Can you work these out from the model? Positions are in its coordinate system, mm. A direction names the side the tool comes from. Round coordinates to 2 decimals unless told otherwise and drop trailing zeros. Loops run counter-clockwise (first coordinate to the right, second up) from the corner with the lowest first, then second, coordinate; pieces in that order, holes last. Notation, with made-up numbers: M 47,60.25 L 85,60.25 A12 ccw 85,68.25 Z; hole C -2.75,46.25 d9. An arc over 180 degrees is marked long. Return JSON: item names as keys, results as strings.
```python
from build123d import *

# Parameters (mm, degrees)
SKETCH3_W                       = 80
SKETCH3_H                       = 80
SKETCH3_W_2                     = 60
SKETCH3_H_2                     = 60
BOSS_EXTRUDE2_DEPTH             = 1550
SKETCH7_W                       = 60
SKETCH7_H                       = 60
BOSS_EXTRUDE3_DEPTH             = 5
BOSS_EXTRUDE4_REACH             = 1561.207
SKETCH8_W                       = 60
SKETCH8_H                       = 5
BOSS_EXTRUDE4_DIRECTION_2_REACH = 1561.207
CUT_EXTRUDE1_REACH              = 1562.929
CUT_EXTRUDE2_REACH              = 1562.929
FILLET1_R                       = 5
MIRROR1_START                   = -90
MIRROR1_DEPTH                   = 10
MIRROR1_2_DEPTH                 = 10
MIRROR1_START_2                 = -80
MIRROR1_3_OUTLINE_W             = 5
MIRROR1_3_OUTLINE_H             = 25
MIRROR1_3_DEPTH                 = 80
MIRROR1_START_3                 = 10
MIRROR1_4_DEPTH                 = 31.124
MIRROR1_START_4                 = -119.452
MIRROR1_5_DEPTH                 = 29.452
MIRROR1_START_5                 = -140
MIRROR1_6_DEPTH                 = 200
MIRROR1_7_DEPTH                 = 5
FILLET1_OF_MIRROR2_R            = 5


with BuildPart() as part:
    # Sketch3 → Boss-Extrude2 (new body)
    with BuildSketch(Plane(origin=(0, 0, 0), x_dir=(0, 0, -1), z_dir=(1, 0, 0))):
        with Locations((40, 40)):
            Rectangle(SKETCH3_W, SKETCH3_H)
        with Locations((40, 40)):
            Rectangle(SKETCH3_W_2, SKETCH3_H_2, mode=Mode.SUBTRACT)
    extrude(amount=BOSS_EXTRUDE2_DEPTH)

    # Sketch7 → Boss-Extrude3 (add)
    with BuildSketch(Plane(origin=(1535, 0, 0), x_dir=(0, 0, -1), z_dir=(1, 0, 0))):
        Polygon((-60, 95), (140, 95), (140, 15), (90, -25), (-10, -25), (-60, 15), align=None)
        with Locations((40, 40)):
            Rectangle(SKETCH7_W, SKETCH7_H, mode=Mode.SUBTRACT)
    boss_extrude3 = extrude(amount=BOSS_EXTRUDE3_DEPTH)

    # Boss-Extrude4: up to this face of the body (flat: up to its plane)
    boss_extrude4_end = Plane(part.part.faces().sort_by_distance((1537.5, 55, -140))[0])
    # Sketch8 → Boss-Extrude4 (add, up to the picked face)
    with BuildSketch(Plane(origin=(0, 0, -80), x_dir=(-1, 0, 0), z_dir=(0, 0, -1)), mode=Mode.PRIVATE) as boss_extrude4_sk1:
        with Locations((-1510, 92.5)):
            Rectangle(SKETCH8_W, SKETCH8_H)
    boss_extrude4_tool1 = split(extrude(boss_extrude4_sk1.sketch, amount=BOSS_EXTRUDE4_REACH, mode=Mode.PRIVATE), bisect_by=boss_extrude4_end, keep=Keep.BOTH, mode=Mode.PRIVATE)
    boss_extrude4 = boss_extrude4_tool1.solids().sort_by(Axis((1510, 92.5, -80), (0, 0, -1)))[0]
    add(boss_extrude4)

    # Boss-Extrude4 direction 2: up to this face of the body (flat: up to its plane)
    boss_extrude4_direction_2_end = Plane(part.part.faces().sort_by_distance((1537.5, 55, 60))[0])
    # Sketch8 → Boss-Extrude4 direction 2 (add, up to the picked face)
    with BuildSketch(Plane(origin=(0, 0, -80), x_dir=(-1, 0, 0), z_dir=(0, 0, -1)), mode=Mode.PRIVATE) as boss_extrude4_direction_2_sk1:
        with Locations((-1510, 92.5)):
            Rectangle(SKETCH8_W, SKETCH8_H)
    boss_extrude4_direction_2_tool1 = split(extrude(boss_extrude4_direction_2_sk1.sketch, amount=-BOSS_EXTRUDE4_DIRECTION_2_REACH, mode=Mode.PRIVATE), bisect_by=boss_extrude4_direction_2_end, keep=Keep.BOTH, mode=Mode.PRIVATE)
    boss_extrude4_direction_2 = boss_extrude4_direction_2_tool1.solids().sort_by(Axis((1510, 92.5, -80), (0, 0, 1)))[0]
    add(boss_extrude4_direction_2)

    # Sketch9 → Cut-Extrude1 (cut, up to next)
    with BuildSketch(Plane(origin=(0, 95, 0), x_dir=(1, 0, 0), z_dir=(0, 1, 0)), mode=Mode.PRIVATE) as cut_extrude1_sk1:
        with BuildLine():
            Line((1480, 80), (1485.801257358, 71.298113962))
            ThreePointArc((1485.801257358, 71.298113962), (1488.927300662, 64.675212774), (1490, 57.430609057))
            Line((1490, 57.430609057), (1490, 22.569390943))
            ThreePointArc((1490, 22.569390943), (1488.927300662, 15.324787226), (1485.801257358, 8.701886038))
            Line((1485.801257358, 8.701886038), (1480, 0))
            Line((1480, 0), (1480, 80))
        make_face()
    cut_extrude1_tool1 = extrude(cut_extrude1_sk1.sketch, amount=-CUT_EXTRUDE1_REACH, mode=Mode.PRIVATE) & part.part
    cut_extrude1 = cut_extrude1_tool1.solids().sort_by_distance((1484.537596, 95, -40))[0]
    add(cut_extrude1, mode=Mode.SUBTRACT)

    # Sketch10 → Cut-Extrude2 (cut, up to next)
    with BuildSketch(Plane(origin=(0, 95, 0), x_dir=(1, 0, 0), z_dir=(0, 1, 0)), mode=Mode.PRIVATE) as cut_extrude2_sk1:
        with BuildLine():
            Line((1500, 126.5), (1520, 126.5))
            ThreePointArc((1520, 126.5), (1526.5, 120), (1520, 113.5))
            Line((1520, 113.5), (1500, 113.5))
            ThreePointArc((1500, 113.5), (1493.5, 120), (1500, 126.5))
        make_face()
    cut_extrude2_tool1 = extrude(cut_extrude2_sk1.sketch, amount=-CUT_EXTRUDE2_REACH, mode=Mode.PRIVATE) & part.part
    # Sketch10 → Cut-Extrude2 (cut, up to next)
    with BuildSketch(Plane(origin=(0, 95, 0), x_dir=(1, 0, 0), z_dir=(0, 1, 0)), mode=Mode.PRIVATE) as cut_extrude2_sk2:
        with BuildLine():
            Line((1500, -33.5), (1520, -33.5))
            ThreePointArc((1520, -33.5), (1526.5, -40), (1520, -46.5))
            Line((1520, -46.5), (1500, -46.5))
            ThreePointArc((1500, -46.5), (1493.5, -40), (1500, -33.5))
        make_face()
    cut_extrude2_tool2 = extrude(cut_extrude2_sk2.sketch, amount=-CUT_EXTRUDE2_REACH, mode=Mode.PRIVATE) & part.part
    cut_extrude2_1 = cut_extrude2_tool1.solids().sort_by_distance((1510, 95, -120))[0]
    add(cut_extrude2_1, mode=Mode.SUBTRACT)
    cut_extrude2_2 = cut_extrude2_tool2.solids().sort_by_distance((1510, 95, 40))[0]
    add(cut_extrude2_2, mode=Mode.SUBTRACT)
    cut_extrude2 = cut_extrude2_1 + cut_extrude2_2  # Cut-Extrude2 as one shape, for the pattern or mirror that repeats it

    # Fillet1
    fillet1_edges = [part.edges().sort_by_distance(p)[0] for p in [
        (1540, 95, -40),
    ]]
    fillet(fillet1_edges, radius=FILLET1_R)

    # Mirror1: read off the stored shape, not the designer's step
    # Mirror1 outline → Mirror1 (add)
    with BuildSketch(Plane.XY.offset(MIRROR1_START)):
        with BuildLine():
            Line((10, 90), (10, -25))
            Line((10, -25), (15, -25))
            Line((15, -25), (15, 95))
            ThreePointArc((15, 95), (11.464466094, 93.535533906), (10, 90))
        make_face()
    extrude(amount=MIRROR1_DEPTH)

    # Mirror1 2 outline → Mirror1 2 (add)
    with BuildSketch(Plane.XY):
        with BuildLine():
            Line((10, 90), (10, -25))
            Line((10, -25), (15, -25))
            Line((15, -25), (15, 95))
            ThreePointArc((15, 95), (11.464466094, 93.535533906), (10, 90))
        make_face()
    extrude(amount=MIRROR1_2_DEPTH)

    # Mirror1 3 outline → Mirror1 3 (add)
    with BuildSketch(Plane.XY.offset(MIRROR1_START_2)):
        with Locations((12.5, -12.5)):
            Rectangle(MIRROR1_3_OUTLINE_W, MIRROR1_3_OUTLINE_H)
        with BuildLine():
            Line((10, 90), (10, 80))
            Line((10, 80), (15, 80))
            Line((15, 80), (15, 95))
            ThreePointArc((15, 95), (11.464466094, 93.535533906), (10, 90))
        make_face()
    extrude(amount=MIRROR1_3_DEPTH)

    # Mirror1 4 outline → Mirror1 4 (add)
    with BuildSketch(Plane.XY.offset(MIRROR1_START_3)):
        with BuildLine():
            Line((10, 0), (15, 0))
            Line((15, 0), (15, 95))
            ThreePointArc((15, 95), (11.464466094, 93.535533906), (10, 90))
            Line((10, 90), (10, 0))
        make_face()
    extrude(amount=MIRROR1_4_DEPTH)

    # Mirror1 5 outline → Mirror1 5 (add)
    with BuildSketch(Plane.XY.offset(MIRROR1_START_4)):
        with BuildLine():
            Line((10, 0), (15, 0))
            Line((15, 0), (15, 95))
            ThreePointArc((15, 95), (11.464466094, 93.535533906), (10, 90))
            Line((10, 90), (10, 0))
        make_face()
    extrude(amount=MIRROR1_5_DEPTH)

    # Mirror1 6 outline → Mirror1 6 (add)
    with BuildSketch(Plane.XY.offset(MIRROR1_START_5)):
        with BuildLine():
            Line((10, 90), (10, 80))
            Line((10, 80), (15, 80))
            Line((15, 80), (15, 95))
            ThreePointArc((15, 95), (11.464466094, 93.535533906), (10, 90))
        make_face()
    extrude(amount=MIRROR1_6_DEPTH)

    # Mirror1 7 outline → Mirror1 7 (add)
    with BuildSketch(Plane.YZ.offset(MIRROR1_START_3)):
        Polygon((80, 41.124), (80, 60), (15, 60), (-25, 10), (0, 10), (0, 41.124), align=None)
        Polygon((0, -90), (-25, -90), (15, -140), (80, -140), (80, -119.452), (0, -119.452), align=None)
    extrude(amount=MIRROR1_7_DEPTH)

    # Mirror2: Boss-Extrude3, Boss-Extrude4, Boss-Extrude4 direction 2, Cut-Extrude1, Cut-Extrude2 across plane
    add(boss_extrude3.mirror(Plane(origin=(775, 0, 0), x_dir=(0, 0, 1), z_dir=(1, 0, 0))))
    add(boss_extrude4.mirror(Plane(origin=(775, 0, 0), x_dir=(0, 0, 1), z_dir=(1, 0, 0))))
    add(boss_extrude4_direction_2.mirror(Plane(origin=(775, 0, 0), x_dir=(0, 0, 1), z_dir=(1, 0, 0))))
    add(cut_extrude1.mirror(Plane(origin=(775, 0, 0), x_dir=(0, 0, 1), z_dir=(1, 0, 0))), mode=Mode.SUBTRACT)
    add(cut_extrude2.mirror(Plane(origin=(775, 0, 0), x_dir=(0, 0, 1), z_dir=(1, 0, 0))), mode=Mode.SUBTRACT)

    # Fillet1 of Mirror2
    fillet1_of_mirror2_edges = [part.edges().sort_by_distance(p)[0] for p in [
        (10, 95, -40),
    ]]
    fillet(fillet1_of_mirror2_edges, radius=FILLET1_OF_MIRROR2_R)


solid = part.part
```
Q1. I'm going to push flat-ended pins straight in: pin 1 Ø8 at (y, z) = (35, 38.5) entering from +X; pin 2 Ø10 at (x, y) = (1102, 11) entering from -Z; pin 3 Ø2 at (x, z) = (743.5, -1) entering from -Y. Where does each tip first touch, or does it pass through?
Results:
{"pin 1": "stops at x = 1540", "pin 2": "stops at z = -80", "pin 3": "stops at y = 0"}
Q2. Thinking about a two-plate mould opening in Y: for faces 1 (the flat face through (764, 10, -40)), 2 (the flat face through (43, 95, -39)), 3 (the flat face through (1537, 70, 60)), which applies, pulls with the +Y half, pulls with the -Y half, needs draft (parallel to the pull), parting line crosses it, or undercut?
Results:
{"face 1": "undercut", "face 2": "pulls with the +Y half", "face 3": "needs draft"}
Q3. If I drill on line 1 along X through (y, z) = (-17, -12.5); line 2 along Z through (x, y) = (809.5, 52.5); line 3 along Y through (x, z) = (1001, -54), over which ranges is the centre line in solid material (lowest first)?
Results:
{"line 1": "x = 10 to 15, 1535 to 1540", "line 2": "z = -80 to -70, -10 to 0", "line 3": "y = 0 to 10, 70 to 80"}
Q4. On a 3-axis mill with a long thin cutter (end or side, diameter ignored), from which of +Z, -Z, +X, -X, +Y, -Y can I reach the whole of each face in a straight line? I mean faces 4 (the flat face through (13, 73, -140)), 5 (the flat face through (764, 70, -40)), 6 (the flat face through (1507, 95, -39)), 7 (the flat face through (42, 90, -41)), 8 (the flat face through (764, 0, -39)). Say none if no direction works.
Results:
{"face 4": "-Z, +X, -X, +Y, -Y", "face 5": "+X, -X", "face 6": "+Z, -Z, +X, -X, +Y", "face 7": "+Z, -Z", "face 8": "+Z, -Z, -Y"}
Q5. Suppose I cut it at A-A, the plane x = 403.5. Please give me the cut outline in (y, z), plus the area to 3 significant figures.
Results:
{"outline": "M 0,-80 L 80,-80 L 80,0 L 0,0 Z; hole M 10,-70 L 70,-70 L 70,-10 L 10,-10 Z", "area": "2,800 mm2"}
Q6. Suppose I cut it at B-B, the plane y = 40. Please give me the cut outline in (x, z).
Results:
{"outline": "M 0,-80 L 10,-80 L 10,-140 L 15,-140 L 15,-80 L 1535,-80 L 1535,-140 L 1540,-140 L 1540,-80 L 1550,-80 L 1550,-70 L 0,-70 Z; M 0,-10 L 1550,-10 L 1550,0 L 1540,0 L 1540,60 L 1535,60 L 1535,0 L 15,0 L 15,60 L 10,60 L 10,0 L 0,0 Z"}
